Geometry: final body of the model. Coordinates: model frame, mm. A direction names the side the tool comes from. Round coordinates to 2 decimals unless told otherwise and drop trailing zeros. Loops run counter-clockwise (first coordinate to the right, second up) from the corner with the lowest first, then second, coordinate; pieces in that order, holes last. Notation, with made-up numbers: M 50,84.5 L 54,84.5 A11 ccw 54,99.5 Z; hole C 72.25,34.25 d8. An arc over 180 degrees is marked long. Write each question's results on one line, items separated by ' | '.
Autodesk Inventor part; units mm, degrees
ref_plane "YZ Plane" through (0, 0, 0) normal (1, 0, 0) x (0, 1, 0)
ref_plane "XZ Plane" through (0, 0, 0) normal (0, 1, 0) x (-1, 0, 0)
ref_plane "XY Plane" through (0, 0, 0) normal (0, 0, 1) x (1, 0, 0)
sketch "Sketch1" plane through (0, 0, 0) normal (0, 1, 0) x (-1, 0, 0)
  point P0 (0, 0)
sketch "Sketch2" plane through (0, 0, 0) normal (0, 1, 0) x (-1, 0, 0)
  point P0 (0, 0)
sketch "Sketch3" plane through (0, 0, 0) normal (0, 1, 0) x (-1, 0, 0)
  line L0 (0, 0) -> (140, 0)
  line L1 (140, 0) -> (140, -100)
  line L2 (140, -100) -> (0, -100)
  line L3 (0, -100) -> (0, 0)
  dimension "d0" = 140
  dimension "d1" = 100
extrude "Extrusion1" add sketch "Sketch3" along normal blind 65
sketch "Sketch4" plane through (0, 0, 0) normal (1, 0, 0) x (0, 0, -1)
  line L0 (3.2517, 3.335) -> (97.2996, 3.335)
  line L1 (97.2996, 3.335) -> (97.2996, 24.6792)
  line L2 (97.2996, 24.6792) -> (3.2517, 24.6792)
  line L3 (3.2517, 24.6792) -> (3.2517, 3.335)
  point P0 (0, 0)
extrude "Extrusion2" cut sketch "Sketch4" against normal blind 136.85
sketch "Sketch6" plane through (0, 0, 0) normal (1, 0, 0) x (0, 0, -1)
  line L0 (3.2517, 32.5271) -> (97.2996, 32.5271)
  line L1 (97.2996, 32.5271) -> (97.2996, 48.6393)
  line L2 (97.2996, 48.6393) -> (3.2517, 48.6393)
  line L3 (3.2517, 48.6393) -> (3.2517, 32.5271)
  point P0 (0, 0)
extrude "Extrusion4" cut sketch "Sketch6" against normal blind 135.4125
sketch "Sketch7" plane through (0, 0, 0) normal (1, 0, 0) x (0, 0, -1)
  line L0 (3.2517, 52.8064) -> (97.2996, 52.8064)
  line L1 (97.2996, 52.8064) -> (97.2996, 62.7809)
  line L2 (97.2996, 62.7809) -> (3.2517, 62.7809)
  line L3 (3.2517, 62.7809) -> (3.2517, 52.8064)
  point P0 (0, 0)
extrude "Extrusion5" cut sketch "Sketch7" against normal blind 134.85
sketch "Sketch8" plane through (0, 0, 0) normal (1, 0, 0) x (0, 0, -1)
  line L0 (97.2996, 62.7809) -> (97.2996, 52.8064)
  line L1 (3.2517, 52.8064) -> (3.2517, 62.7809)
  line L2 (97.2996, 52.8064) -> (3.2517, 52.8064)
  line L3 (3.2517, 62.7809) -> (97.2996, 62.7809)
  line L4 (97.2996, 32.5271) -> (3.2517, 32.5271)
  line L5 (3.2517, 48.6393) -> (97.2996, 48.6393)
  line L6 (97.2996, 48.6393) -> (97.2996, 32.5271)
  line L7 (3.2517, 32.5271) -> (3.2517, 48.6393)
  line L8 (97.2996, 24.6792) -> (97.2996, 3.335)
  line L9 (3.2517, 3.335) -> (3.2517, 24.6792)
  line L10 (97.2996, 3.335) -> (3.2517, 3.335)
  line L11 (3.2517, 24.6792) -> (97.2996, 24.6792)
  point P0 (0, 0)
  point P1 (3.2517, 57.7937)
  dimension "d20" = 94.048
  dimension "d21" = 9.9745
  dimension "d22" = 16.1122
  dimension "d23" = 94.048
  dimension "d24" = 94.048
  dimension "d25" = 21.3442
sketch "Sketch9" plane through (0, 0, 0) normal (1, 0, 0) x (0, 0, -1)
  line L0 (100, 0) -> (100, 65)
  line L1 (0, 0) -> (0, 65)
  line L2 (0, 0) -> (100, 0)
  line L3 (0, 65) -> (100, 65)
  line L4 (3.2517, 62.7809) -> (97.2996, 62.7809)
  line L5 (3.2517, 52.8064) -> (3.2517, 62.7809)
  line L6 (3.2517, 48.6393) -> (97.2996, 48.6393)
  line L7 (97.2996, 52.8064) -> (3.2517, 52.8064)
  line L8 (3.2517, 32.5271) -> (3.2517, 48.6393)
  line L9 (3.2517, 24.6792) -> (97.2996, 24.6792)
  line L10 (97.2996, 32.5271) -> (3.2517, 32.5271)
  line L11 (97.2996, 48.6393) -> (97.2996, 32.5271)
  line L12 (3.2517, 3.335) -> (3.2517, 24.6792)
  line L13 (97.2996, 24.6792) -> (97.2996, 3.335)
  line L14 (97.2996, 3.335) -> (3.2517, 3.335)
  dimension "d26" = 100
  dimension "d27" = 65
  dimension "d28" = 2.2191
  dimension "d29" = 3.2517
  dimension "d30" = 4.167
  dimension "d31" = 3.2517
  dimension "d32" = 7.8479
  dimension "d33" = 2.7004
  dimension "d34" = 3.2517
  dimension "d35" = 2.7004
  dimension "d36" = 3.335
sketch "Sketch10" plane through (0, 65, 0) normal (0, 1, 0) x (1, 0, 0)
  line L0 (0, 0) -> (0, 100)
  circle A0 centre (0, 51.3457) radius 7.5
  point P0 (0, 58.8457)
  point P1 (0, 43.8457)
  dimension "d37" = 15
extrude "Extrusion6" cut sketch "Sketch10" against normal blind 65 contours A0 L0 picked at (-3.0801, 51.117)
properties part number "hddcase"
1. Access query for faces 1 (the face through (-67, 3.335, -50)), 2 (the face through (-7.5, 28.7, -51.5)). Directions: +Z, -Z, +X, -X, +Y, -Y. A direction counts if a zero-diameter tool reaches every point of the face in a straight line with its end or side. Return the directions, or none.
Answer key:
face 1: +X | face 2: +X, +Y, -Y
2. Ray query, probe 1 along Y at (x, z) = (-124, -59) (3 decimals); probe 2 along Z at (x, y) = (-122, 17.5); probe 3 along X at (y, z) = (19, -34). Return the intervals inside material, ascending.
Answer key:
probe 1: y = 0 to 3.335, 24.679 to 32.527, 48.639 to 52.806, 62.781 to 65 | probe 2: z = -100 to -97.3, -3.25 to 0 | probe 3: x = -140 to -136.85
3. Pin query (flat end, axial travel): P1, Ø5, axis at y = 55.5, z = -68.5, coming from the +X side. Return the tip coordinate at first contact, or that it passes through.
Answer key:
P1: stops at x = -134.85
4. Section A-A (x = -129). Output: boundary loops of the cut face in (y, z) (3 decimals).
Answer key:
outline: M 0,-100 L 65,-100 L 65,0 L 0,0 Z; hole M 3.335,-97.3 L 24.679,-97.3 L 24.679,-3.252 L 3.335,-3.252 Z; hole M 32.527,-97.3 L 48.639,-97.3 L 48.639,-3.252 L 32.527,-3.252 Z; hole M 52.806,-97.3 L 62.781,-97.3 L 62.781,-3.252 L 52.806,-3.252 Z
